Answer from the drawing. Dimensions are ordinates in mm from the lowest x, y and z of the part. Coordinates: 2 decimals unless noted, no trailing zeros. Order: outer loops, then holes, each group sorted by start corner. A loop starts at its lowest first (then second) coordinate and runs counter-clockwise, first axis right, second up. Notation, with made-up numbers: (23.5, 88) -> (35.5, 88) arc R17 cw to (35.5, 111) -> close; hole circle Ø3 at (58.25, 4.5). An arc over 180 degrees is marked (long way). Answer in a Markdown table with one row per item.
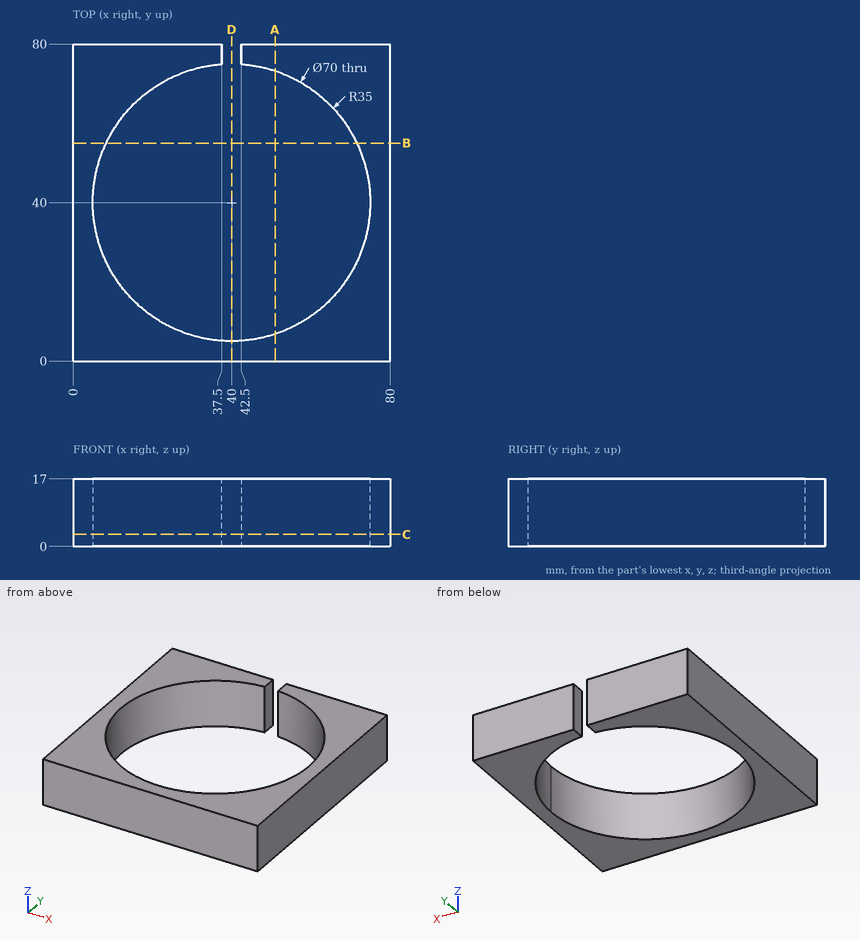
(1) Find the intervals of material crossed by line 1 along X through (y, z) = (40, 5.75); line 2 along Y through (x, z) = (40, 13.5); line 3 along X through (y, z) = (76.5, 14), in increasing order. Write a range as from..to.
Check values:
| item | result |
|---|---|
| line 1 | 0..5, 75..80 |
| line 2 | 0..5 |
| line 3 | 0..37.5, 42.5..80 |
(2) A cutting plane is placed at A-A, the plane x = 51. Determine the outline of the cut face in (y, z).
Check values:
| item | result |
|---|---|
| outline | (0, 0) -> (6.77, 0) -> (6.77, 17) -> (0, 17) -> close; (73.23, 0) -> (80, 0) -> (80, 17) -> (73.23, 17) -> close |
(3) A cutting plane is placed at B-B, the plane y = 55. Determine the outline of the cut face in (x, z).
Check values:
| item | result |
|---|---|
| outline | (0, 0) -> (8.38, 0) -> (8.38, 17) -> (0, 17) -> close; (71.62, 0) -> (80, 0) -> (80, 17) -> (71.62, 17) -> close |
(4) A cutting plane is placed at D-D, the plane x = 40. Determine the outline of the cut face in (y, z).
Check values:
| item | result |
|---|---|
| outline | (0, 0) -> (5, 0) -> (5, 17) -> (0, 17) -> close |
(5) A cutting plane is placed at C-C, the plane z = 3. Determine the outline of the cut face in (x, y), then the cut area to 3 significant figures.
Check values:
| item | result |
|---|---|
| outline | (0, 0) -> (80, 0) -> (80, 80) -> (42.5, 80) -> (42.5, 74.91) arc R35 cw (long way) to (37.5, 74.91) -> (37.5, 80) -> (0, 80) -> close |
| area | 2,530 mm² |
